Design review of the part built by this model. Coordinates are the model's own, in mm. Face numbers are marked on the shaded views. A direction names the side the tool comes from. Coordinates: 2 decimals unless noted, no trailing zeros. Order: outer loops, then holes, each group sorted by start corner. A loop starts at its lowest first (then second) coordinate and runs counter-clockwise, first axis right, second up. Notation, with made-up numbers: M -25,19 L -1,19 A31 cw -1,51 Z; hole C 9,38 d2. An arc over 180 degrees is marked long. Use CSV: the item, a comma, the result in double quotes.
```python
from build123d import *

# Parameters (mm, degrees)
SKETCH_1_R          = 14
EXTRUDE_1_DEPTH     = 34
SKETCH_2_R          = 2.75
EXTRUDE_2_DEPTH     = 10
SKETCH_3_R          = 7.6
CUT_EXTRUDE_1_DEPTH = 45
CHAMFER_1_SIZE      = 0.5


with BuildPart() as part:
    # Эскиз1 → Бобышка-Вытянуть1 (new body)
    with BuildSketch(Plane(origin=(0, 0, 0), x_dir=(1, 0, 0), z_dir=(0, 1, 0))):
        Circle(SKETCH_1_R)
    extrude(amount=EXTRUDE_1_DEPTH)

    # Эскиз2 → Бобышка-Вытянуть2 (add)
    with BuildSketch(Plane(origin=(0, 34, 0), x_dir=(1, 0, 0), z_dir=(0, 1, 0))):
        with BuildLine():
            Line((-20.25, -12.881673028), (-20.25, 12.881673028))
            ThreePointArc((-20.25, 12.881673028), (0, 24), (20.25, 12.881673028))
            Line((20.25, 12.881673028), (20.25, -12.881673028))
            ThreePointArc((20.25, -12.881673028), (0, -24), (-20.25, -12.881673028))
        make_face()
        with Locations((0, 19)):
            Circle(SKETCH_2_R, mode=Mode.SUBTRACT)
        with Locations((13.435028843, 13.435028843)):
            Circle(SKETCH_2_R, mode=Mode.SUBTRACT)
        with Locations((13.435028843, -13.435028843)):
            Circle(SKETCH_2_R, mode=Mode.SUBTRACT)
        with Locations((0, -19)):
            Circle(SKETCH_2_R, mode=Mode.SUBTRACT)
        with Locations((-13.435028843, -13.435028843)):
            Circle(SKETCH_2_R, mode=Mode.SUBTRACT)
        with Locations((-13.435028843, 13.435028843)):
            Circle(SKETCH_2_R, mode=Mode.SUBTRACT)
    extrude(amount=EXTRUDE_2_DEPTH)

    # Эскиз3 → Вырез-Вытянуть1 (cut, through all)
    with BuildSketch(Plane(origin=(0, 44, 0), x_dir=(1, 0, 0), z_dir=(0, 1, 0))):
        Circle(SKETCH_3_R)
    extrude(amount=-CUT_EXTRUDE_1_DEPTH, mode=Mode.SUBTRACT)

    # Фаска1
    chamfer_1_edges = [part.edges().sort_by_distance(p)[0] for p in [
        (-14, 0, 0),
        (0, 44, -24),
        (-20.25, 44, 0),
        (0, 44, 24),
        (20.25, 44, 0),
        (0, 34, -24),
        (-20.25, 34, 0),
        (0, 34, 24),
        (20.25, 34, 0),
    ]]
    chamfer(chamfer_1_edges, length=CHAMFER_1_SIZE)


solid = part.part
```
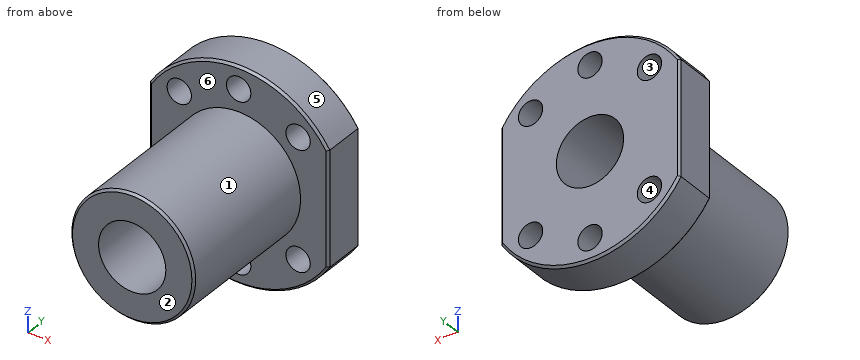
(1) Wall thickness on probe 1 along Z at (x, y) = (0, 37); probe 2 along Z at (x, y) = (2.5, 36.5); probe 3 along X at (y, z) = (39.5, 14): over which ranges is each line inside the solid? List them lowest first.
The answers:
probe 1,"z = -24 to -21.75, -16.25 to -7.6, 7.6 to 16.25, 21.75 to 24"
probe 2,"z = -23.87 to -20.15, -17.85 to -7.18, 7.18 to 17.85, 20.15 to 23.87"
probe 3,"x = -19.49 to -16.13, -10.74 to 10.74, 16.13 to 19.49"
(2) Add section C-C on y = 37.5. State the section outline as (x, z) points.
The answers:
outline,"M -20.25,-12.88 A24 ccw 20.25,-12.88 L 20.25,12.88 A24 ccw -20.25,12.88 Z; hole C -13.44,-13.44 d5.5; hole C -13.44,13.44 d5.5; hole C 0,0 d15.2; hole C 0,-19 d5.5; hole C 0,19 d5.5; hole C 13.44,-13.44 d5.5; hole C 13.44,13.44 d5.5"
(3) Add section B-B on z = 0. State the section outline as (x, y) points, and give its area (3 significant figures).
The answers:
outline,"M -20.25,34.5 L -19.75,34 L -14,34 L -14,0.5 L -13.5,0 L -7.6,0 L -7.6,44 L -19.75,44 L -20.25,43.5 Z; M 7.6,0 L 13.5,0 L 14,0.5 L 14,34 L 19.75,34 L 20.25,34.5 L 20.25,43.5 L 19.75,44 L 7.6,44 Z"
area,"687 mm2"
(4) Add section A-A on x = 0. State the section outline as (y, z) points, and give its area (3 significant figures).
The answers:
outline,"M 0,-13.5 L 0.5,-14 L 34,-14 L 34,-16.25 L 44,-16.25 L 44,-7.6 L 0,-7.6 Z; M 0,7.6 L 44,7.6 L 44,16.25 L 34,16.25 L 34,14 L 0.5,14 L 0,13.5 Z; M 34,-23.5 L 34.5,-24 L 43.5,-24 L 44,-23.5 L 44,-21.75 L 34,-21.75 Z; M 34,21.75 L 44,21.75 L 44,23.5 L 43.5,24 L 34.5,24 L 34,23.5 Z"
area,"652 mm2"
(5) Add section D-D on y = 18. State the section outline as (x, z) points, and give its area (3 significant figures).
The answers:
outline,"C 0,0 d28; hole C 0,0 d15.2"
area,"434 mm2"
(6) Clearance check with flat-ended pins moving along their axes: P1, Ø12, axis at y = 10, z = -3, coming from the -X side; P2, Ø9, axis at x = 0, z = 0, coming from the +Y side; P3, Ø6.5, axis at x = 0, z = -19, coming from the -Y side; P4, Ø7, axis at x = 13.44, z = -13.44, coming from the +Y side. State where each tip first meets the part, or that it passes through.
The answers:
P1,"stops at x = -14"
P2,"passes through"
P3,"stops at y = 34"
P4,"stops at y = 44"
(7) The part is to be moulded in two halves that separate along X. For the marked faces 3, 4, 5 and 6, say which applies: pulls with the +X half, pulls with the -X half, needs draft (parallel to the pull), parting line crosses it, or undercut.
The answers:
face 3,"undercut"
face 4,"undercut"
face 5,"parting line crosses it"
face 6,"needs draft"
(8) For the marked faces 1 and 2, list the 3-axis set-ups (+Z, -Z, +X, -X, +Y, -Y) from which the entire face can be reached by the end or side of a thin tool; tool diameter is ignored.
The answers:
face 1,"-Y"
face 2,"+Z, -Z, +X, -X, -Y"
